CAD build for the part. Positions are in the model's coordinates, mm. Coordinates: 2 decimals unless noted, no trailing zeros. Write each loop counter-clockwise with the first axis right and the second up, starting at its lowest first coordinate (ties: lowest second). Pieces come first, ordered by that corner, then holes. Notation, with made-up numbers: (45, -8.75) - (85, -8.75) arc R6 ccw to (85, 0.25) - close; hole circle Ø2 at (88, 87). An arc over 180 degrees is marked (long way). Answer in a Markdown table with one row per item. Add a question column.
Q1. Drill centre lines: line 1 along X through (y, z) = (-237.5, 2.4) (3 decimals); line 2 along Y through (x, z) = (45, 2.45); line 3 along Y through (x, z) = (-76.5, 0.55). Where is each one in solid material? Low to high. Write a range as from..to.
Q2. Band-saw the part on C-C (z = 1.55). State how many separate pieces and enclosed holes the cut face has, and give its area (3 significant figures).
Q3. Two-plate mould, pull along X, no slides. Class faces 1 (the flat face through (-1, -3, 3.175)), 2 (the cylindrical face through (40.8, 65.8, 1.6)): +X half, -X half, draft (parallel to the pull), parting line (faces both ways), or undercut.
Q4. Band-saw the part on A-A (y = -76). List the corners of the cut face in (x, z) (3 decimals), and give its area (3 significant figures).
Q5. Pin check, flat tip, straight feed: pin 1 (3.5 mm diameter, centred on x = 69.915, y = -237.5, fed in from +Z). Stop position of the tip, or through.
Q6. Band-saw the part on B-B (x = 37). List the corners of the cut face in (y, z) (3 decimals).
```python
from build123d import *

# Parameters (mm, degrees)
SKETCH1_W           = 500
SKETCH1_H           = 171.83
SKETCH1_R           = 1.7
SKETCH1_R_2         = 28
SKETCH1_R_3         = 2.8
SKETCH1_R_4         = 3.5
BOSS_EXTRUDE1_DEPTH = 3.175
SKETCH2_W           = 171.83
SKETCH2_H           = 500
SKETCH2_W_2         = 170.83
SKETCH2_H_2         = 499
CUT_EXTRUDE1_DEPTH  = 3.175


with BuildPart() as part:
    # Sketch1 → Boss-Extrude1 (new body)
    with BuildSketch(Plane(origin=(0, 0, 0), x_dir=(0, 1, 0), z_dir=(0, 0, 1))):
        Rectangle(SKETCH1_W, SKETCH1_H)
        with Locations(Location((57.42, -45.305, 0), (0, 0, 270))):
            Circle(SKETCH1_R, mode=Mode.SUBTRACT)
        with Locations(Location((30.382686894, 1.525, 0), (0, 0, 270))):
            Circle(SKETCH1_R, mode=Mode.SUBTRACT)
        with Locations(Location((84.457313106, 1.525, 0), (0, 0, 270))):
            Circle(SKETCH1_R, mode=Mode.SUBTRACT)
        with Locations(Location((145.212686894, 1.525, 0), (0, 0, 270))):
            Circle(SKETCH1_R, mode=Mode.SUBTRACT)
        with Locations(Location((-57.42, -45.305, 0), (0, 0, 270))):
            Circle(SKETCH1_R, mode=Mode.SUBTRACT)
        with Locations(Location((-30.382686894, 1.525, 0), (0, 0, 270))):
            Circle(SKETCH1_R, mode=Mode.SUBTRACT)
        with Locations(Location((-145.212686894, 1.525, 0), (0, 0, 270))):
            Circle(SKETCH1_R, mode=Mode.SUBTRACT)
        with Locations(Location((-199.287313106, 1.525, 0), (0, 0, 270))):
            Circle(SKETCH1_R, mode=Mode.SUBTRACT)
        with Locations(Location((-172.25, -45.305, 0), (0, 0, 270))):
            Circle(SKETCH1_R, mode=Mode.SUBTRACT)
        with Locations(Location((172.25, -14.085, 0), (0, 0, 270))):
            Circle(SKETCH1_R_2, mode=Mode.SUBTRACT)
        with Locations(Location((-57.42, -14.085, 0), (0, 0, 270))):
            Circle(SKETCH1_R_2, mode=Mode.SUBTRACT)
        with Locations(Location((-172.25, -14.085, 0), (0, 0, 270))):
            Circle(SKETCH1_R_2, mode=Mode.SUBTRACT)
        with Locations(Location((237.5, -69.915, 0), (0, 0, 270))):
            Circle(SKETCH1_R_3, mode=Mode.SUBTRACT)
        with Locations(Location((-237.5, -69.915, 0), (0, 0, 270))):
            Circle(SKETCH1_R_3, mode=Mode.SUBTRACT)
        with Locations(Location((237.5, 73.415, 0), (0, 0, 270))):
            Circle(SKETCH1_R_4, mode=Mode.SUBTRACT)
        with Locations(Location((-237.5, 73.415, 0), (0, 0, 270))):
            Circle(SKETCH1_R_4, mode=Mode.SUBTRACT)
        with Locations(Location((57.42, -14.085, 0), (0, 0, 270))):
            Circle(SKETCH1_R_2, mode=Mode.SUBTRACT)
        with Locations(Location((-84.457313106, 1.525, 0), (0, 0, 270))):
            Circle(SKETCH1_R, mode=Mode.SUBTRACT)
        with Locations(Location((199.287313106, 1.525, 0), (0, 0, 270))):
            Circle(SKETCH1_R, mode=Mode.SUBTRACT)
        with Locations(Location((172.25, -45.305, 0), (0, 0, 270))):
            Circle(SKETCH1_R, mode=Mode.SUBTRACT)
    extrude(amount=BOSS_EXTRUDE1_DEPTH)

    # Sketch2 → Cut-Extrude1 (cut)
    with BuildSketch(Plane.XY.offset(3.175)):
        Rectangle(SKETCH2_W, SKETCH2_H)
        Rectangle(SKETCH2_W_2, SKETCH2_H_2, mode=Mode.SUBTRACT)
    extrude(amount=-CUT_EXTRUDE1_DEPTH, mode=Mode.SUBTRACT)


solid = part.part
```
Checked values:
| question | item | result |
|---|---|---|
| 1 | line 1 | x = -85.415..-76.915, -69.915..67.115, 72.715..85.415 |
| 1 | line 2 | y = -249.5..-173.92, -170.58..-59.09, -55.75..55.75, 59.09..170.58, 173.92..249.5 |
| 1 | line 3 | y = -249.5..-239.15, -235.85..235.85, 239.15..249.5 |
| 2 | separate pieces | 1 |
| 2 | enclosed holes | 20 |
| 2 | area | 75,200 mm² |
| 3 | face 1 | draft |
| 3 | face 2 | undercut |
| 4 | outline | (-85.415, 0) - (-6.862, 0) - (-6.862, 3.175) - (-85.415, 3.175) - close; (35.032, 0) - (85.415, 0) - (85.415, 3.175) - (35.032, 3.175) - close |
| 4 | area | 409 mm² |
| 5 | pin 1 | passes through |
| 6 | outline | (-249.5, 0) - (-188.34, 0) - (-188.34, 3.175) - (-249.5, 3.175) - close; (-156.16, 0) - (-73.51, 0) - (-73.51, 3.175) - (-156.16, 3.175) - close; (-41.33, 0) - (41.33, 0) - (41.33, 3.175) - (-41.33, 3.175) - close; (73.51, 0) - (156.16, 0) - (156.16, 3.175) - (73.51, 3.175) - close; (188.34, 0) - (249.5, 0) - (249.5, 3.175) - (188.34, 3.175) - close |
